```python
from build123d import *

# Parameters (mm, degrees)
PAD_DEPTH       = 80
THICKNESS_T     = 5
SKETCH002_R     = 11
SKETCH002_R_2   = 2.5
POCKET001_DEPTH = 5
SKETCH003_W     = 300
SKETCH003_H     = 15
POCKET002_DEPTH = 5
SKETCH004_W     = 729.94403
SKETCH004_H     = 312.833175
POCKET_DEPTH    = 5
SKETCH005_R     = 3
HOLE_DEPTH      = 25
SKETCH006_R     = 12.5
POCKET003_DEPTH = 5


with BuildPart() as part:
    # Sketch → Pad (new body)
    with BuildSketch(Plane.XY):
        with BuildLine():
            Line((275, 0), (275, 60))
            ThreePointArc((275, 60), (260.355339, 95.355339), (225, 110))
            Line((225, 110), (-225, 110))
            ThreePointArc((-225, 110), (-260.355339, 95.355339), (-275, 60))
            Line((-275, 60), (-275, 0))
            Line((-275, 0), (275, 0))
        make_face()
    extrude(amount=PAD_DEPTH)

    # Thickness
    thickness_openings = [part.faces().sort_by_distance(p)[0] for p in [
        (0, 0, 40),
    ]]
    offset(amount=THICKNESS_T, openings=thickness_openings)

    # Sketch002 → Pocket001 (cut)
    with BuildSketch(Plane.XY.offset(85)):
        with Locations((-200, 50)):
            Circle(SKETCH002_R)
        with Locations((-150, 50)):
            Circle(SKETCH002_R)
        with Locations((-245, 60)):
            Circle(SKETCH002_R_2)
        with Locations((245, 60)):
            Circle(SKETCH002_R_2)
    extrude(amount=-POCKET001_DEPTH, mode=Mode.SUBTRACT)

    # Sketch003 (on Face15 of Pocket001) → Pocket002 (cut)
    with BuildSketch(Plane.XZ.offset(-110)):
        with Locations((-10, 47.5)):
            Rectangle(SKETCH003_W, SKETCH003_H)
    extrude(amount=-POCKET002_DEPTH, mode=Mode.SUBTRACT)

    # Sketch004 (on Face10 of Pocket002) → Pocket (cut)
    with BuildSketch(Plane(origin=(0, 0, -5), x_dir=(1, 0, 0), z_dir=(0, 0, -1))):
        with Locations((-35.610138, -20.133613)):
            Rectangle(SKETCH004_W, SKETCH004_H)
    extrude(amount=-POCKET_DEPTH, mode=Mode.SUBTRACT)

    # Sketch005 (on Face9 of Pocket) → Hole (cut)
    with BuildSketch(Plane.XY.offset(85)):
        with Locations((-75, 60)):
            Circle(SKETCH005_R)
        with Locations((-60, 60)):
            Circle(SKETCH005_R)
        with Locations((60, 60)):
            Circle(SKETCH005_R)
        with Locations((75, 60)):
            Circle(SKETCH005_R)
    extrude(amount=-HOLE_DEPTH, mode=Mode.SUBTRACT)

    # Sketch006 (on Face9 of Hole) → Pocket003 (cut)
    with BuildSketch(Plane.XY.offset(85)):
        with Locations((0, 53.851604)):
            Circle(SKETCH006_R)
    extrude(amount=-POCKET003_DEPTH, mode=Mode.SUBTRACT)


solid = part.part
```
Source: CAD feature listing. Evaluate the final solid. Frame: model axes, mm. A direction names the side the tool comes from. Coordinates: 2 decimals unless noted, no trailing zeros. Loops run counter-clockwise (first coordinate to the right, second up) from the corner with the lowest first, then second, coordinate; pieces in that order, holes last. Notation, with made-up numbers: M 81.25,41 L 120.25,41 A25 cw 120.25,58 Z; hole C 14,-11 d3. An arc over 180 degrees is marked long. Put each result on its own line as item: value. Start each with the question number.
1) Reachability of faces 5 (the face through (-275, 30, 39)), 6 (the face through (-263.461, 99.316, 39.44)) from +Z, -Z, +X, -X, +Y, -Y: full face, straight path, thin tool, end or side. Return the list, or none.
2) Contact query for flat-ended pins moving along their axis: pin 1 Ø6 at (y, z) = (67, 38) entering from +X; pin 2 Ø24 at (x, z) = (-24, 53.5) entering from -Y; pin 3 Ø9.5 at (x, y) = (75, 60) entering from -Z; pin 4 Ø5.5 at (x, y) = (-70, 112) entering from +Z. Output: stop coordinate, or through.
3) Ray query, L1, parallel to X at y = 44.5, z = 59; L2, parallel to Z at x = 0, y = 80; L3, parallel to X at y = 94, z = 25.5. Return the intervals inside material, ascending. Write a range as from..to.
4) Cut plane A-A on x = 130.5. Return the cut outline in (y, z).
5) Cut plane D-D on y = 7.5. Return the cut outline in (x, z).
6) Cut plane C-C on z = 26. Return the cut outline in (x, y), then the cut area to 3 significant figures.
7) Pull-direction query (X, two-part tool) for faces 1 (the face through (-211, 50, 83)), 2 (the face through (-4, 68, 80)), 3 (the face through (-280, 30, 39)), 4 (the face through (264.316, 98.461, 39.44)); classes: pulls with the +X half, pulls with the -X half, needs draft (parallel to the pull), parting line crosses it, or undercut.
8) Cut plane B-B on x = -150. Return the cut outline in (y, z).
The answers:
1. face 5: -Z, -Y
1. face 6: +Z, -Z, -X, +Y
2. pin 1: stops at x = 279.85
2. pin 2: stops at y = 110
2. pin 3: stops at z = 80
2. pin 4: stops at z = 85
3. L1: x = -280..-275, 275..280
3. L2: z = 80..85
3. L3: x = -268.23..-261.66, 261.66..268.23
4. outline: M 0,80 L 110,80 L 110,55 L 115,55 L 115,80 A5 ccw 110,85 L 0,85 Z; M 110,0 L 115,0 L 115,40 L 110,40 Z
5. outline: M -280,0 L -275,0 L -275,80 L 275,80 L 275,0 L 280,0 L 280,80 A5 ccw 275,85 L -275,85 A5 ccw -280,80 Z
6. outline: M -280,0 L -275,0 L -275,60 A50 cw -225,110 L 225,110 A50 cw 275,60 L 275,0 L 280,0 L 280,60 A55 ccw 225,115 L -225,115 A55 ccw -280,60 Z
6. area: 3,670 mm²
7. face 1: undercut
7. face 2: undercut
7. face 3: pulls with the -X half
7. face 4: pulls with the +X half
8. outline: M 0,80 L 39,80 L 39,85 L 0,85 Z; M 61,80 L 110,80 L 110,55 L 115,55 L 115,80 A5 ccw 110,85 L 61,85 Z; M 110,0 L 115,0 L 115,40 L 110,40 Z
